Build history of the part. All positions in model axes, mm. A direction names the side the tool comes from. Round coordinates to 2 decimals unless told otherwise and drop trailing zeros. Write each loop counter-clockwise with the first axis right and the second up, starting at its lowest first coordinate (ties: lowest second). Pieces come first, ordered by that corner, then holes. Notation, with made-up numbers: M 51.25,-18.75 L 74.25,-18.75 A13 ccw 74.25,-5.75 Z; hole C -34.75,-1.5 d7. An arc over 180 degrees is marked long. Write item = value, one per line. Start each with the question number.
Q1. Band-saw the part on D-D on y = 28.5. Write the cut outline in (x, z).
Q2. Band-saw the part on C-C on z = 19.05. Write the cut outline in (x, y).
Q3. Drop flat-ended pins along their axis: P1, Ø4, axis at x = 12.7, z = 19.05, coming from the +Y side; P2, Ø2, axis at x = 8, z = 32.5, coming from the +Y side; P3, Ø3, axis at y = 11, z = 9, coming from the +X side; P4, Ø8, axis at x = 6.5, z = 21, coming from the +Y side. Give the stop position or say it passes through.
Q4. Pull direction X, two halves, no side cores. Call faces 6 (the cylindrical face through (12.38, 2.41, 16.58)), 7 (the cylindrical face through (1.21, 30.88, 19.12)), 8 (the flat face through (2.381, 31, 21)): released by +X, released by -X, zero draft, split by the parting line, or undercut.
Q5. Probe L1, parallel to Z at x = 12.7, y = 3.4; L2, parallel to Y at x = 10.25, z = 35. List the from-to ranges inside material, lowest first.
Q6. Band-saw the part on A-A on z = 6.35. Write the cut outline in (x, y), plus the area to 3 significant figures.
Q7. Band-saw the part on B-B on x = 12.7. Write the cut outline in (y, z), plus the area to 3 significant figures.
Q8. Tool access for faces 1 (the cylindrical face through (18.1, 2.35, 0.91)), 2 (the cylindrical face through (3.589, 27.786, 19.281)), 3 (the cylindrical face through (2.35, 50.16, 25.59)), 4 (the cylindrical face through (10.213, 2.415, 6.241)), 5 (the flat face through (4.762, 23, 19)): list every direction of +Z, -Z, +X, -X, +Y, -Y with a clear straight run to the whole face (end or side of a thin tool).
Autodesk Inventor part; units mm, degrees
ref_plane "YZ Plane" through (0, 0, 0) normal (1, 0, 0) x (0, 1, 0)
ref_plane "XZ Plane" through (0, 0, 0) normal (0, 1, 0) x (-1, 0, 0)
ref_plane "XY Plane" through (0, 0, 0) normal (0, 0, 1) x (1, 0, 0)
sketch "Sketch2" plane through (0, 0, 0) normal (0, 0, 1) x (1, 0, 0)
  line L0 (0, 0) -> (0, 50.8)
  line L1 (0, 50.8) -> (4.7625, 50.8)
  line L2 (4.7625, 50.8) -> (4.7625, 4.7625)
  line L3 (4.7625, 4.7625) -> (19.05, 4.7625)
  line L4 (19.05, 4.7625) -> (19.05, 0)
  line L5 (19.05, 0) -> (0, 0)
  dimension "d0" = 4.7625
  dimension "d1" = 50.8
  dimension "d2" = 19.05
extrude "Extrusion1" add sketch "Sketch2" along normal blind 38.1
sketch "Sketch3" plane through (4.7625, 4.7625, 0) normal (1, 0, 0) x (0, 0, -1)
  circle A0 centre (-19.05, 29.3688) radius 3.2512
  line L0 (-22.3012, 29.3688) -> (-22.3012, 35.7188)
  line L1 (-22.3012, 35.7188) -> (-25.0661, 46.0375)
  line L2 (0, 46.0375) -> (-38.1, 46.0375)
  line L3 (-13.0339, 46.0375) -> (-15.7988, 35.7188)
  line L4 (-15.7988, 35.7188) -> (-15.7988, 29.3688)
  line L5 (-38.1, 0) -> (-38.1, 46.0375)
  point P0 (0, -4.7625)
  point P1 (-19.05, 46.0375)
  point P2 (-38.1, 23.0187)
  point P3 (-38.1, 23.0187)
  dimension "d5" = 6.5024
  dimension "d6" = 165
  dimension "d7" = 6.35
  dimension "d18" = 6.35
extrude "Extrusion2" cut sketch "Sketch3" against normal blind 38.1
sketch "Sketch4" plane through (4.7625, 4.7625, 0) normal (0, 1, 0) x (1, 0, 0)
  circle A0 centre (7.9375, -31.75) radius 2.4892
  circle A1 centre (7.9375, -6.35) radius 2.4892
  line L0 (14.2875, -38.1) -> (0, -38.1)
  line L1 (14.2875, 0) -> (0, 0)
  circle A2 centre (7.9375, -19.05) radius 2.4892
  line L2 (-4.7625, -25.0661) -> (-4.7625, -38.1)
  point P0 (-4.7625, 0)
  point P1 (7.1437, -38.1)
  dimension "d10" = 4.9784
  dimension "d11" = 4.9784
  dimension "d12" = 6.35
  dimension "d13" = 6.35
  dimension "d14" = 25.4
  dimension "d22" = 12.7
  dimension "d23" = 12.7
extrude "Extrusion3" cut sketch "Sketch4" against normal blind 38.1
fillet "Fillet1" radius 3.175 6 edges at (2.3813, 50.8, 38.1) (2.3813, 50.8, 25.0661) (2.3813, 50.8, 13.0339) (2.3813, 50.8, 0) (19.05, 2.3813, 38.1) (19.05, 2.3813, 0)
sketch "Sketch5" plane through (4.7625, 4.7625, 38.1) normal (1, 0, 0) x (0, 0, -1)
  arc A0 (15.7988, 29.3688) -> (22.3012, 29.3688) centre (19.05, 29.3688) ccw
  circle A1 centre (19.05, 29.3688) radius 6.35
  point P0 (38.1, -4.7625)
  dimension "d19" = 12.7
extrude "Extrusion4" cut sketch "Sketch5" against normal blind 2.3813
equation "\"d13\" = d12"
properties part number "BUMP_007_Smallbracket" material "Aluminum 6061"
Conclusion:
q1.outline = M 0,0 L 4.76,0 L 4.76,16.12 L 2.38,16.12 L 2.38,21.98 L 4.76,21.98 L 4.76,38.1 L 0,38.1 Z
q2.outline = M 0,0 L 10.21,0 L 10.21,4.76 L 4.76,4.76 L 4.76,27.78 L 2.38,27.78 L 2.38,30.88 L 0,30.88 Z; M 15.19,0 L 19.05,0 L 19.05,4.76 L 15.19,4.76 Z
q3.P1 = through
q3.P2 = 4.76
q3.P3 = 4.76
q3.P4 = 48.92
q4.face_6 = undercut
q4.face_7 = zero draft
q4.face_8 = released by +X
q5.L1 = 0 to 3.86, 8.84 to 16.56, 21.54 to 29.26, 34.24 to 38.1
q5.L2 = 0 to 4.76
q6.outline = M 0,0 L 10.21,0 L 10.21,4.76 L 4.76,4.76 L 4.76,50.8 L 0,50.8 Z; M 15.19,0 L 19.05,0 L 19.05,4.76 L 15.19,4.76 Z
q6.area = 286 mm^2
q7.outline = M 0,0 L 4.76,0 L 4.76,3.86 L 0,3.86 Z; M 0,8.84 L 4.76,8.84 L 4.76,16.56 L 0,16.56 Z; M 0,21.54 L 4.76,21.54 L 4.76,29.26 L 0,29.26 Z; M 0,34.24 L 4.76,34.24 L 4.76,38.1 L 0,38.1 Z
q7.area = 110 mm^2
q8.face_1 = -Z, +X, +Y, -Y
q8.face_2 = +X
q8.face_3 = +X, -X, +Y
q8.face_4 = +Y, -Y
q8.face_5 = +Z, -Z, +X, +Y
